The listing builds one solid part. Answer for the finished solid, in the listing's coordinates (mm). Coordinates: 2 decimals unless noted, no trailing zeros.
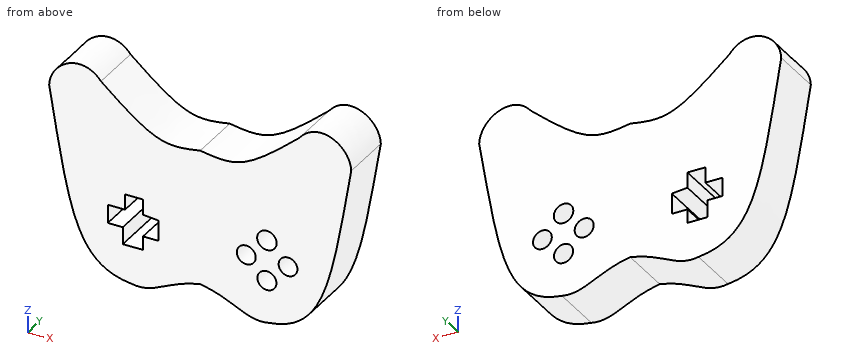
from build123d import *

# Parameters (mm, degrees)
SKETCH1_R           = 0.358119717
SKETCH1_R_2         = 0.367977628
SKETCH1_R_3         = 0.354400667
SKETCH1_R_4         = 0.360009999
BOSS_EXTRUDE1_DEPTH = 2


with BuildPart() as part:
    # Sketch1 → Boss-Extrude1 (new body)
    with BuildSketch(Plane(origin=(0, 0, 0), x_dir=(1, 0, 0), z_dir=(0, 1, 0))):
        with BuildLine():
            add(Edge.make_bspline(
                [(9.515794057, 8.168972603), (8.277051231, 8.384166889), (7.783662178, 9.075903216), (6.938322746, 8.906835329)],
                knots=[0, 0, 0, 0, 1, 1, 1, 1], degree=3))
            add(Edge.make_bspline(
                [(6.938322746, 8.906835329), (4.786223752, 8.676253294), (4.567934499, 6.637882364), (3.814703871, 2.179986806)],
                knots=[0, 0, 0, 0, 1, 1, 1, 1], degree=3))
            add(Edge.make_bspline(
                [(3.814703871, 2.179986806), (3.85569383, 1.237217744), (5.062947097, 0.587465173), (5.770040096, 1.479017216)],
                knots=[0, 0, 0, 0, 1, 1, 1, 1], degree=3))
            add(Edge.make_bspline(
                [(5.770040096, 1.479017216), (7.783771597, 3.231424782), (8.154064913, 3.299063972), (9.515794057, 3.053124366)],
                knots=[0, 0, 0, 0, 1, 1, 1, 1], degree=3))
            add(Edge.make_bspline(
                [(13.261548017, 1.479017216), (11.247816516, 3.231424782), (10.8775232, 3.299063972), (9.515794057, 3.053124366)],
                knots=[0, 0, 0, 0, 1, 1, 1, 1], degree=3))
            add(Edge.make_bspline(
                [(15.216884243, 2.179986806), (15.175894283, 1.237217744), (13.968641017, 0.587465173), (13.261548017, 1.479017216)],
                knots=[0, 0, 0, 0, 1, 1, 1, 1], degree=3))
            add(Edge.make_bspline(
                [(12.093265367, 8.906835329), (14.245364361, 8.676253294), (14.463653614, 6.637882364), (15.216884243, 2.179986806)],
                knots=[0, 0, 0, 0, 1, 1, 1, 1], degree=3))
            add(Edge.make_bspline(
                [(9.515794057, 8.168972603), (10.754536882, 8.384166889), (11.247925935, 9.075903216), (12.093265367, 8.906835329)],
                knots=[0, 0, 0, 0, 1, 1, 1, 1], degree=3))
        make_face()
        with Locations((11.254257148, 6.545084301)):
            Circle(SKETCH1_R, mode=Mode.SUBTRACT)
        with Locations((12.032572113, 5.766769337)):
            Circle(SKETCH1_R_2, mode=Mode.SUBTRACT)
        with Locations((12.830512487, 6.545084301)):
            Circle(SKETCH1_R_3, mode=Mode.SUBTRACT)
        with Locations((12.032572113, 7.306018511)):
            Circle(SKETCH1_R_4, mode=Mode.SUBTRACT)
        Polygon((6.680070792, 7.480300725), (7.356444958, 7.480300725), (7.356444958, 6.963796816), (7.946735139, 6.963796816), (7.946735139, 6.189040953), (7.356444958, 6.133334516), (7.356444958, 5.549559924), (6.680070792, 5.549559924), (6.680070792, 6.133334516), (6.02829205, 6.133334516), (6.02829205, 6.831056674), (6.593986807, 6.831056674), (6.593986807, 7.480300725), align=None, mode=Mode.SUBTRACT)
    extrude(amount=BOSS_EXTRUDE1_DEPTH)


solid = part.part
1. Section A-A on y = 0.5 is taken. State how many separate pieces and enclosed holes the cut face has, then the cut area to 3 significant figures.
Results found:
separate pieces: 1
enclosed holes: 5
area: 60.8 mm2
2. Flat-ended cylindrical pins translate along their axes: P1, Ø0.6, axis at y = 1, z = -6, coming from the -X side; P2, Ø1, axis at y = 1.5, z = -5.5, coming from the +X side; P3, Ø1, axis at y = 1, z = -7.5, coming from the -X side; P4, Ø0.5, axis at x = 7, y = 1, coming from the -Z side. Find the tip coordinate at first contact, or state that the pin passes through.
Results found:
P1: stops at x = 4.45
P2: stops at x = 14.73
P3: stops at x = 4.8
P4: stops at z = -8.93
3. Find the intervals of material crossed by L1, parallel to X at y = 0.35, z = -6; L2, parallel to Z at x = 11.75, y = 1; L3, parallel to X at y = 0.35, z = -6.75, in increasing order.
Results found:
L1: x = 4.52 to 6.68, 7.36 to 11.75, 12.32 to 14.52
L2: z = -8.93 to -7.53, -7.08 to -6, -5.53 to -2.69
L3: x = 4.72 to 6.03, 7.95 to 10.96, 11.55 to 12.54, 13.12 to 14.31
